```python
from build123d import *

# Parameters (mm, degrees)
CROQUIS1_R              = 1.25
SALIENTE_EXTRUIR1_DEPTH = 1
SALIENTE_EXTRUIR2_DEPTH = 6
CORTAR_EXTRUIR1_DEPTH   = 22
SALIENTE_EXTRUIR3_DEPTH = 3
CROQUIS5_W              = 2.5
CROQUIS5_H              = 3
SALIENTE_EXTRUIR4_DEPTH = 2.5


with BuildPart() as part:
    # Croquis1 → Saliente-Extruir1 (new body)
    with BuildSketch(Plane(origin=(0, 0, 0), x_dir=(1, 0, 0), z_dir=(0, 1, 0))):
        with BuildLine():
            Line((-11.5, -10.5), (11.5, -10.5))
            ThreePointArc((11.5, -10.5), (13.267766953, -9.767766953), (14, -8))
            Line((14, -8), (14, 8))
            ThreePointArc((14, 8), (13.267766953, 9.767766953), (11.5, 10.5))
            Line((11.5, 10.5), (-11.5, 10.5))
            ThreePointArc((-11.5, 10.5), (-13.267766953, 9.767766953), (-14, 8))
            Line((-14, 8), (-14, -8))
            ThreePointArc((-14, -8), (-13.267766953, -9.767766953), (-11.5, -10.5))
        make_face()
        with Locations(Location((11.75, -8.25, 0), (0, 0, 270))):
            Circle(CROQUIS1_R, mode=Mode.SUBTRACT)
        with Locations(Location((11.75, 8.25, 0), (0, 0, 270))):
            Circle(CROQUIS1_R, mode=Mode.SUBTRACT)
        with Locations(Location((-11.75, 6.25, 0), (0, 0, 270))):
            Circle(CROQUIS1_R, mode=Mode.SUBTRACT)
        with Locations(Location((-11.75, -6.25, 0), (0, 0, 270))):
            Circle(CROQUIS1_R, mode=Mode.SUBTRACT)
    extrude(amount=SALIENTE_EXTRUIR1_DEPTH)

    # Croquis2 → Saliente-Extruir2 (add)
    with BuildSketch(Plane(origin=(0, 1, 0), x_dir=(1, 0, 0), z_dir=(0, 1, 0))):
        Polygon((14, -3.5), (6, -3.5), (6, -2.5), (7.5, -2.5), (7.5, 2.5), (6, 2.5), (6, 3.5), (14, 3.5), align=None)
    extrude(amount=SALIENTE_EXTRUIR2_DEPTH)

    # Croquis3 → Cortar-Extruir1 (cut, through all)
    with BuildSketch(Plane.XY.offset(3.5)):
        Polygon((7.5, 7), (7.5, 5.064017175), (6, 4), (6, 7), align=None)
    extrude(amount=-CORTAR_EXTRUIR1_DEPTH, mode=Mode.SUBTRACT)

    # Croquis4 → Saliente-Extruir3 (add)
    with BuildSketch(Plane(origin=(0, 1, 0), x_dir=(1, 0, 0), z_dir=(0, 1, 0))):
        Polygon((-3, -5.5), (0, -5.5), (1, -4.5), (1, -1.5), (0, -0.5), (-3, -0.5), (-4, -1.5), (-4, -4.5), align=None)
    extrude(amount=SALIENTE_EXTRUIR3_DEPTH)

    # Croquis5 → Saliente-Extruir4 (add)
    with BuildSketch(Plane(origin=(0, 1, 0), x_dir=(1, 0, 0), z_dir=(0, 1, 0))):
        with Locations((-4.75, 7.5)):
            Rectangle(CROQUIS5_W, CROQUIS5_H)
    extrude(amount=SALIENTE_EXTRUIR4_DEPTH)


solid = part.part
```
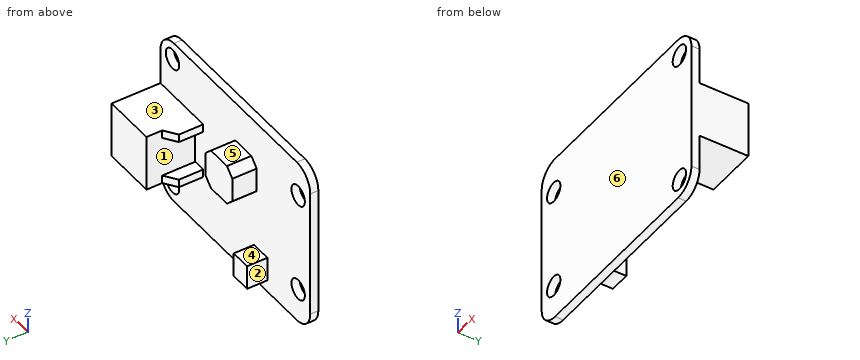
Can you work these out from the model? Positions are in its coordinate system, mm. Face numbers are marked on the shaded views. A direction names the side the tool comes from. Coordinates: 2 decimals unless noted, no trailing zeros. Loops run counter-clockwise (first coordinate to the right, second up) from the corner with the lowest first, then second, coordinate; pieces in that order, holes last. Notation, with made-up numbers: (-38.75, 21.25) - (13.25, 21.25) arc R18 cw to (13.25, 51.25) - close; hole circle Ø1 at (-22, 37). An arc over 180 degrees is marked (long way). Use a Markdown table: item, result.
Item 1: I want a section at C-C on z = 6.25. Please give me the cut outline in (x, y), and give its area (3 significant figures).
Numbers:
| item | result |
|---|---|
| outline | (-14, 0) - (-13, 0) - (-13, 1) - (-14, 1) - close; (-10.5, 0) - (14, 0) - (14, 1) - (-10.5, 1) - close |
| area | 25.5 mm2 |
Item 2: I want a section at D-D on x = -4.75. Please give me the cut outline in (y, z).
Numbers:
| item | result |
|---|---|
| outline | (0, -10.5) - (1, -10.5) - (1, -9) - (3.5, -9) - (3.5, -6) - (1, -6) - (1, 10.5) - (0, 10.5) - close |
Item 3: For the marked faces 1, 2 and 3, which set-ups out of +Z, -Z, +X, -X, +Y, -Y let a thin tool reach every point of the face, with its end or its side?
Numbers:
| item | result |
|---|---|
| face 1 | +Y |
| face 2 | +Z, -Z, -X, +Y |
| face 3 | +Z, +X, +Y |
Item 4: We'd pull the mould along Z, two halves only. Please class the marked faces 4, 5 and 6: released by +Z, released by -Z, zero draft, split by the parting line, or undercut.
Numbers:
| item | result |
|---|---|
| face 4 | undercut |
| face 5 | released by +Z |
| face 6 | zero draft |
Item 5: I want a section at B-B on x = 11. Please give me the cut outline in (y, z).
Numbers:
| item | result |
|---|---|
| outline | (0, -10.5) - (1, -10.5) - (1, -9.25) - (0, -9.25) - close; (0, -7.25) - (1, -7.25) - (1, -3.5) - (7, -3.5) - (7, 3.5) - (1, 3.5) - (1, 7.25) - (0, 7.25) - close; (0, 9.25) - (1, 9.25) - (1, 10.5) - (0, 10.5) - close |
Item 6: If I drill on probe 1 along X at (y, z) = (0.3, 6.25); probe 2 along Y at (x, z) = (10, -7.5); probe 3 along Z at (x, y) = (11, 5.25), over which ranges is the centre line in solid material (lowest first)? Write a range as from..to.
Numbers:
| item | result |
|---|---|
| probe 1 | x = -14..-13, -10.5..14 |
| probe 2 | y = 0..1 |
| probe 3 | z = -3.5..3.5 |
Item 7: I want a section at A-A on y = 3. Please give me the cut outline in (x, z).
Numbers:
| item | result |
|---|---|
| outline | (-6, -9) - (-3.5, -9) - (-3.5, -6) - (-6, -6) - close; (-4, 1.5) - (-3, 0.5) - (0, 0.5) - (1, 1.5) - (1, 4.5) - (0, 5.5) - (-3, 5.5) - (-4, 4.5) - close; (6, -3.5) - (14, -3.5) - (14, 3.5) - (6, 3.5) - (6, 2.5) - (7.5, 2.5) - (7.5, -2.5) - (6, -2.5) - close |
Item 8: Will these pins go through, and if not, where does the flat tip stop? pin 1 (3 mm diameter, centred on x = 11, y = 3.5, fed in from +Z); pin 2 (1 mm diameter, centred on x = 0.5, z = -6, fed in from +Y); pin 3 (5.5 mm diameter, centred on x = -0.5, z = 3.5, fed in from +Y).
Numbers:
| item | result |
|---|---|
| pin 1 | stops at z = 3.5 |
| pin 2 | stops at y = 1 |
| pin 3 | stops at y = 4 |
